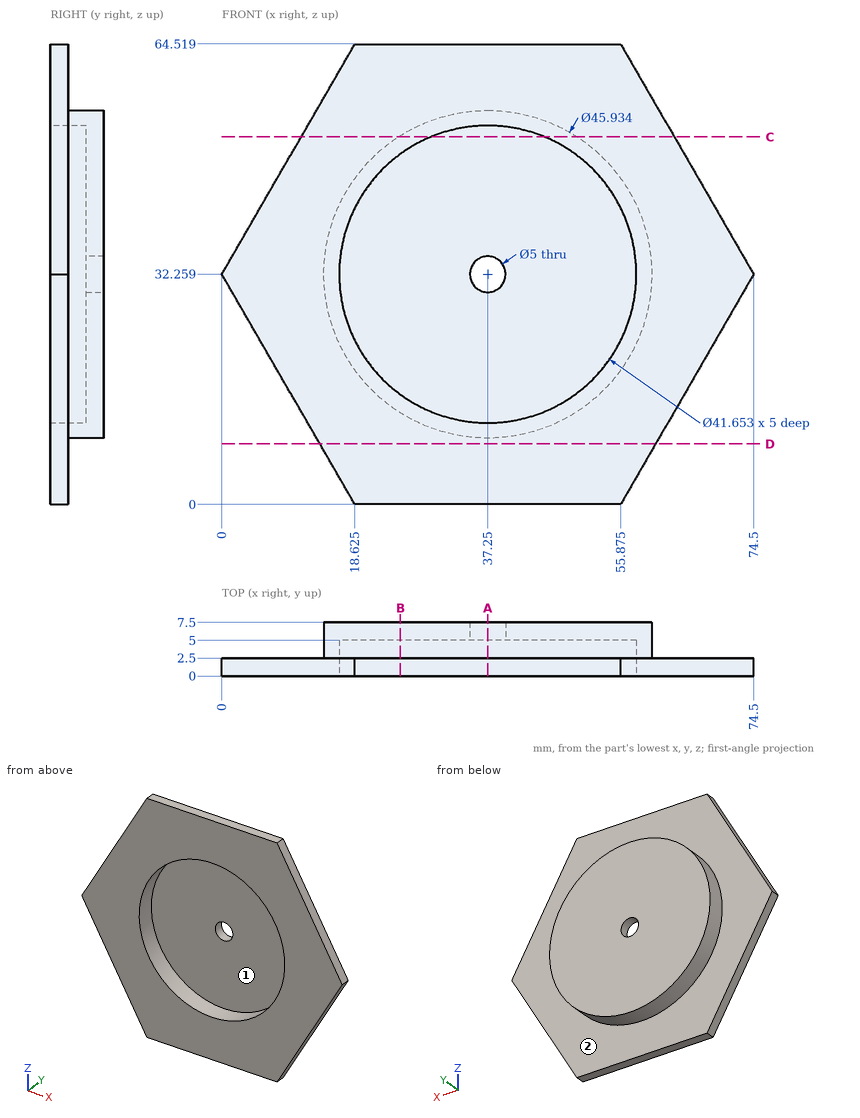
Print and shaded views of the part. All mm, measured from the part's lowest x, y and z. Round coordinates to 2 decimals unless told otherwise and drop trailing zeros. Write each loop counter-clockwise with the first axis right and the second up, starting at its lowest first coordinate (ties: lowest second). Pieces come first, ordered by that corner, then holes. Notation, with made-up numbers: (66.5, -0.5) - (84.5, -0.5) arc R23 cw to (84.5, 12.5) - close; hole circle Ø1 at (-21.75, 39.25). An arc over 180 degrees is marked (long way). One line per item, written item: value.
(1) Cut at C-C, the plane z = 51.5. Give the cut face in (x, y).
Values follow:
outline: (11.11, 0) - (29.28, 0) - (29.28, 5) - (45.22, 5) - (45.22, 0) - (63.39, 0) - (63.39, 2.5) - (49.79, 2.5) - (49.79, 7.5) - (24.71, 7.5) - (24.71, 2.5) - (11.11, 2.5) - close
(2) Wall check: probe 1 along X at (y, z) = (2.25, 22) (1 decimal); probe 2 along Z at (x, y) = (28.5, 0.5); probe 3 along X at (y, z) = (4.5, 44.5) (1 decimal). Give the ranges that are in metal, low to high.
Values follow:
probe 1: x = 5.9 to 19.1, 55.4 to 68.6
probe 2: z = 0 to 13.36, 51.16 to 64.52
probe 3: x = 17.8 to 20.4, 54.1 to 56.7
(3) Cut at A-A, the plane x = 37.25. Give the cut face in (y, z).
Values follow:
outline: (0, 0) - (2.5, 0) - (2.5, 9.29) - (7.5, 9.29) - (7.5, 29.76) - (5, 29.76) - (5, 11.43) - (0, 11.43) - close; (0, 53.09) - (5, 53.09) - (5, 34.76) - (7.5, 34.76) - (7.5, 55.23) - (2.5, 55.23) - (2.5, 64.52) - (0, 64.52) - close
(4) Drop flat-ended pins along their axis: P1, Ø21, axis at x = 42.5, z = 25, coming from the -Y side; P2, Ø4, axis at y = 5, z = 10, coming from the +X side; P3, Ø2, axis at y = 3, z = 16.5, coming from the +X side. Give the stop position or say it passes through.
Values follow:
P1: stops at y = 5
P2: stops at x = 48.07
P3: stops at x = 65.9
(5) Cut at B-B, the plane x = 25. Give the cut face in (y, z), plus the area to 3 significant figures.
Values follow:
outline: (0, 0) - (2.5, 0) - (2.5, 12.83) - (7.5, 12.83) - (7.5, 51.69) - (2.5, 51.69) - (2.5, 64.52) - (0, 64.52) - (0, 49.1) - (5, 49.1) - (5, 15.42) - (0, 15.42) - close
area: 187 mm²
(6) Two-plate mould, pull along X, no slides. Class the marked faces 1 and 2: pulls with the +X half, pulls with the -X half, needs draft (parallel to the pull), parting line crosses it, or undercut.
Values follow:
face 1: undercut
face 2: needs draft
(7) Cut at D-D, the plane z = 8.5. Give the cut face in (x, y).
Values follow:
outline: (13.72, 0) - (60.78, 0) - (60.78, 2.5) - (13.72, 2.5) - close
